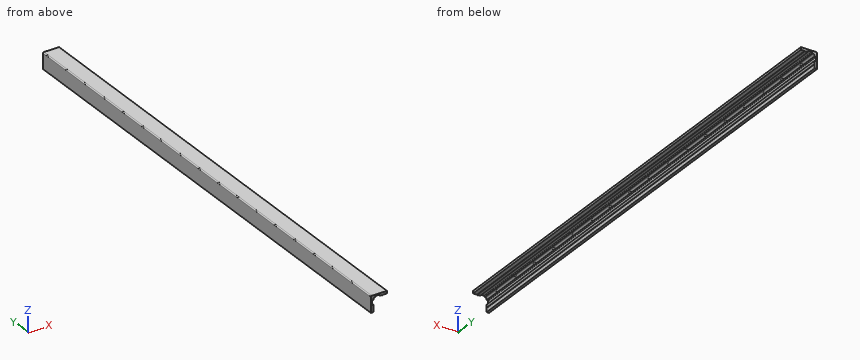
```python
from build123d import *

# Parameters (mm, degrees)
BOSS_EXTRUDE1_DEPTH = 1828.8
SKETCH6_W           = 1
SKETCH6_H           = 4
BOSS_EXTRUDE2_DEPTH = 1828.8
SKETCH7_W           = 4
SKETCH7_H           = 1
BOSS_EXTRUDE3_DEPTH = 1828.8
SKETCH8_W           = 15.75
SKETCH8_H           = 4.5
CUT_EXTRUDE3_DEPTH  = 1829.8
SKETCH9_W           = 4.5
SKETCH9_H           = 15.75
CUT_EXTRUDE4_DEPTH  = 1829.8
FILLET4_R           = 2
FILLET2_R           = 3.66
FILLET3_R           = 3.66


with BuildPart() as part:
    # Sketch2 → Boss-Extrude1 (new body)
    with BuildSketch(Plane(origin=(0, 0, 0), x_dir=(1, 0, 0), z_dir=(0, 1, 0))):
        Polygon((0, 0), (50, 0), (50, -9), (-9, -9), (-9, 50), (0, 50), align=None)
    extrude(amount=BOSS_EXTRUDE1_DEPTH)

    # Sketch6 → Boss-Extrude2 (add, through all)
    with BuildSketch(Plane(origin=(0, 1828.8, 0), x_dir=(1, 0, 0), z_dir=(0, 1, 0))):
        with Locations((0.5, 33.75)):
            Rectangle(SKETCH6_W, SKETCH6_H)
    extrude(amount=-BOSS_EXTRUDE2_DEPTH)

    # Sketch7 → Boss-Extrude3 (add, through all)
    with BuildSketch(Plane(origin=(0, 1828.8, 0), x_dir=(1, 0, 0), z_dir=(0, 1, 0))):
        with Locations((33.75, 0.5)):
            Rectangle(SKETCH7_W, SKETCH7_H)
    extrude(amount=-BOSS_EXTRUDE3_DEPTH)

    # Sketch8 → Cut-Extrude3 (cut, through all)
    with BuildSketch(Plane(origin=(0, 1828.8, 0), x_dir=(1, 0, 0), z_dir=(0, 1, 0))):
        with Locations((15.875, -2.25)):
            Rectangle(SKETCH8_W, SKETCH8_H)
    extrude(amount=-CUT_EXTRUDE3_DEPTH, mode=Mode.SUBTRACT)

    # Sketch9 → Cut-Extrude4 (cut, through all)
    with BuildSketch(Plane(origin=(0, 1828.8, 0), x_dir=(1, 0, 0), z_dir=(0, 1, 0))):
        with Locations((-2.25, 15.875)):
            Rectangle(SKETCH9_W, SKETCH9_H)
    extrude(amount=-CUT_EXTRUDE4_DEPTH, mode=Mode.SUBTRACT)

    # Fillet4
    fillet4_edges = [part.edges().sort_by_distance(p)[0] for p in [
        (8, 914.4, 4.5),
        (23.75, 914.4, 4.5),
        (-4.5, 914.4, -8),
        (-4.5, 914.4, -23.75),
    ]]
    fillet(fillet4_edges, radius=FILLET4_R)

    # Fillet2
    fillet2_edges = [part.edges().sort_by_distance(p)[0] for p in [
        (0, 914.4, 0),
    ]]
    fillet(fillet2_edges, radius=FILLET2_R)

    # Fillet3
    fillet3_edges = [part.edges().sort_by_distance(p)[0] for p in [
        (-9, 914.4, 9),
    ]]
    fillet(fillet3_edges, radius=FILLET3_R)


solid = part.part
```
Part model, mm, in its own coordinate system. Coordinates: 2 decimals unless noted, no trailing zeros. Order: outer loops, then holes, each group sorted by start corner. A loop starts at its lowest first (then second) coordinate and runs counter-clockwise, first axis right, second up. Notation, with made-up numbers: (-12, -6) - (37, -6) arc R25 cw to (37, 30) - close; hole circle Ø9 at (-30, 62). An arc over 180 degrees is marked (long way). Return JSON: item names as keys, results as strings. Group by question number.
Item 1: Cut at A-A (y = 282.5). List the corners of the cut face in (x, z), plus the area to 3 significant figures.
Item 2: Drill centre lines: probe 1 along X at (y, z) = (983, 1); probe 2 along X at (y, z) = (878.5, -39); probe 3 along Z at (x, y) = (21, 1587.5). Where is each one in solid material? Low to high. Write a range as from..to.
Item 3: Pin check, flat tips, straight feed: pin 1 (9 mm diameter, centred on y = 970, z = -29.5, fed in from +X); pin 2 (6 mm diameter, centred on x = 14.5, y = 1585.5, fed in from -Z); pin 3 (7 mm diameter, centred on y = 984.5, z = -41, fed in from +X). Stop position of each tip, or through.
Check values:
{
 "1": {"outline": "(-9, -50) - (0, -50) - (0, -35.75) - (1, -35.75) - (1, -31.75) - (0, -31.75) - (0, -23.75) - (-2.5, -23.75) arc R2 cw to (-4.5, -21.75) - (-4.5, -10) arc R2 cw to (-2.5, -8) - (0, -8) - (0, -3.66) arc R3.66 cw to (3.66, 0) - (8, 0) - (8, 2.5) arc R2 cw to (10, 4.5) - (21.75, 4.5) arc R2 cw to (23.75, 2.5) - (23.75, 0) - (31.75, 0) - (31.75, -1) - (35.75, -1) - (35.75, 0) - (50, 0) - (50, 9) - (-5.34, 9) arc R3.66 ccw to (-9, 5.34) - close", "area": "851 mm2"},
 "2": {"probe 1": "x = -9..8, 23.75..50", "probe 2": "x = -9..0", "probe 3": "z = 4.5..9"},
 "3": {"pin 1": "stops at x = 1", "pin 2": "stops at z = 4.5", "pin 3": "stops at x = 0"}
}
